from build123d import *

# Parameters (mm, degrees)
F1_DEPTH = 7


with BuildPart() as f1:
    # F0 (on Top) → F1 (new body)
    with BuildSketch(Plane.XY):
        with BuildLine():
            Line((31.75, 0), (-31.75, 0))
            ThreePointArc((-31.75, 0), (-34.704196, 6.696799), (-27.766563, 4.363636))
            ThreePointArc((-27.766563, 4.363636), (-26.136411, 3.006211), (-24.778986, 4.636364))
            ThreePointArc((-24.778986, 4.636364), (-36.919843, 8.719399), (-31.75, -3))
            Line((-31.75, -3), (31.75, -3))
            ThreePointArc((31.75, -3), (36.335039, -0.870066), (37.664802, 4.007528))
            ThreePointArc((37.664802, 4.007528), (36.670299, 6.433753), (34.736073, 8.204168))
            ThreePointArc((34.736073, 8.204168), (32.7542, 7.280006), (33.678363, 5.298133))
            ThreePointArc((33.678363, 5.298133), (34.569078, 1.97394), (31.75, 0))
        make_face()
        with BuildLine():
            add(Edge.make_bspline(
                [(37.664802, 4.007528), (38.646857, 0.955298), (43.6282, 0.290702), (46.75, -0.003234)],
                knots=[0.170737, 0.170737, 0.170737, 0.170737, 10.040086, 10.040086, 10.040086, 10.040086], degree=3))
            ThreePointArc((37.664802, 4.007528), (36.335039, -0.870066), (31.75, -3))
            Line((31.75, -3), (46.75, -3))
            ThreePointArc((46.75, -3), (48.248383, -1.501617), (46.75, -0.003234))
        make_face()
    extrude(amount=F1_DEPTH)


solid = f1.part
Check sheet for the modelled part. Datum: model origin and axes. Units: mm. Round coordinates to 2 decimals unless told otherwise and drop trailing zeros. Loops run counter-clockwise (first coordinate to the right, second up) from the corner with the lowest first, then second, coordinate; pieces in that order, holes last.
1. Sectioned sample at C-C on y = -1.5. Record the boundary of the cut face in (x, z), and give its area (3 significant figures).
2. Gauge pin test, flat ends, axial feed: pin 1 Ø8 at (x, y) = (17.5, 7) entering from +Z; pin 2 Ø1.5 at (y, z) = (5, 2.5) entering from +X; pin 3 Ø4 at (y, z) = (0.5, 5) entering from -X. Record the tip position at first contact, or that the pin passes through.
3. Sectioned sample at B-B on x = 17.5. Record the boundary of the cut face in (y, z).
4. Sectioned sample at A-A on x = -26. Record the boundary of the cut face in (y, z).
5. Scan lines: probe 1 along X at (y, z) = (4, 4.5); probe 2 along Y at (x, z) = (-31.75, 5.25); probe 3 along X at (y, z) = (3.75, 6). Record each from-to range of solid material in increasing order.
6. Mould release check, pull along Y, two halves, no side actions. Record for faces 1 (the cylindrical face through (36.691, 6.403, 3.451)), 2 (the cylindrical face through (-36.764, 8.884, 3.451)), 3 (the cylindrical face through (-26.2, 3, 3.5)), 4 (the cylindrical face through (34.586, 2.022, 3.451)): released by +Y, released by -Y, zero draft, split by the parting line, or undercut.
Recorded:
1. outline: (-36.08, 0) - (48.25, 0) - (48.25, 7) - (-36.08, 7) - close
1. area: 590 mm2
2. pin 1: passes through
2. pin 2: stops at x = 37.62
2. pin 3: stops at x = -38.59
3. outline: (-3, 0) - (0, 0) - (0, 7) - (-3, 7) - close
4. outline: (-3, 0) - (0, 0) - (0, 7) - (-3, 7) - close; (3.03, 0) - (7.99, 0) - (7.99, 7) - (3.03, 7) - close
5. probe 1: x = -38.75 to -35.75, -27.69 to -24.86, 34.58 to 37.67
5. probe 2: y = -3 to 0, 8 to 11
5. probe 3: x = -38.75 to -35.74, -27.57 to -24.97, 34.65 to 37.76
6. face 1: released by +Y
6. face 2: split by the parting line
6. face 3: undercut
6. face 4: undercut
